Build history of the part. All positions in model axes, mm. Give positions to 0.01 mm unless a question says otherwise; leave off trailing zeros. Write each loop counter-clockwise with the first axis right and the second up, starting at its lowest first coordinate (ties: lowest second). Pieces come first, ordered by that corner, then holes. Notation, with made-up numbers: (28, -25.5) -> (72, -25.5) arc R8 cw to (72, -20.5) -> close; hole circle Ø5 at (-4.5, 35). An arc over 180 degrees is marked (long way). One line per question, with ' | ' between items. Start each with the question number.
(1) Band-saw the part on A-A, the plane z = 0. Give the cut face in (x, y), and give its area (3 significant figures).
(2) Pin check, flat tips, straight feed: P1, Ø0.9, axis at x = 10, y = 1, coming from the +Z side; P2, Ø0.6, axis at y = 1.5, z = 9, coming from the +X side; P3, Ø1.5, axis at y = 1.5, z = 0, coming from the -X side; P4, Ø1.7, axis at x = -21, z = 32.86, coming from the -Y side. Stop position of each tip, or through.
(3) Band-saw the part on C-C, the plane z = -21. Give the cut face in (x, y).
(4) Band-saw the part on D-D, the plane x = -8.5. Give the cut face in (y, z), and give its area (3 significant figures).
(5) Band-saw the part on B-B, the plane x = -55. Give the cut face in (y, z).
(6) Drill centre lines: probe 1 along X at (y, z) = (0.6, 16); probe 2 along X at (y, z) = (1.6, -18); probe 3 along Z at (x, y) = (31.5, 0.55). Where is each one in solid material? Low to high. Write a range as from..to.
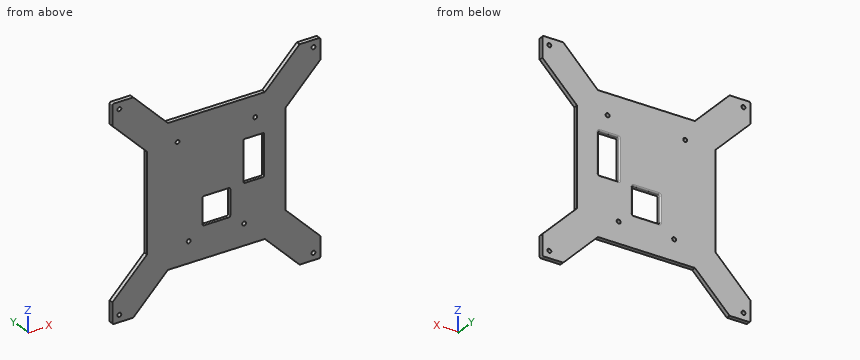
Autodesk Inventor part; units mm, degrees
ref_plane "YZ Plane" through (0, 0, 0) normal (1, 0, 0) x (0, 1, 0)
ref_plane "XZ Plane" through (0, 0, 0) normal (0, 1, 0) x (-1, 0, 0)
ref_plane "XY Plane" through (0, 0, 0) normal (0, 0, 1) x (1, 0, 0)
sketch "Sketch2" plane through (0, 0, 0) normal (0, 1, 0) x (-1, 0, 0)
  line L0 (67.9954, 72.8645) -> (-82.0046, 72.8645)
  line L1 (-82.0046, 72.8645) -> (-82.0046, -77.1355)
  line L2 (-82.0046, -77.1355) -> (67.9954, -77.1355)
  line L3 (67.9954, -77.1355) -> (67.9954, 72.8645)
  circle A0 centre (62.9954, 67.8645) radius 1.4
  line L4 (67.9954, -2.1355) -> (-82.0046, -2.1355)
  line L5 (-7.0046, 72.8645) -> (-7.0046, -77.1355)
  circle A1 centre (62.9954, -72.1355) radius 1.4
  circle A2 centre (-77.0046, 67.8645) radius 1.4
  circle A3 centre (-77.0046, -72.1355) radius 1.4
  point P0 (0, 0)
  dimension "d0" = 150
  dimension "d1" = 150
  dimension "d2" = 5
  dimension "d3" = 5
  dimension "d43" = 2.8
extrude "Extrusion1" add sketch "Sketch2" along normal blind 3
sketch "Sketch4" plane through (0, 3, 0) normal (0, 1, 0) x (1, 0, 0)
  line L0 (-12.9954, 37.1355) -> (27.0046, 37.1355)
  line L1 (27.0046, 37.1355) -> (35.0046, -32.8645)
  line L2 (35.0046, -32.8645) -> (-20.9954, -32.8645)
  line L3 (-20.9954, -32.8645) -> (-12.9954, 37.1355)
  line L4 (7.0046, 37.1355) -> (7.0046, -32.8645)
  line L5 (82.0046, -72.8645) -> (82.0046, 77.1355)
  line L6 (-16.9954, 2.1355) -> (31.0046, 2.1355)
  line L7 (82.0046, 77.1355) -> (-67.9954, 77.1355)
  circle A0 centre (-12.9954, 37.1355) radius 1.4
  circle A1 centre (27.0046, 37.1355) radius 1.4
  circle A2 centre (35.0046, -32.8645) radius 1.4
  circle A3 centre (-20.9954, -32.8645) radius 1.4
  line L8 (26.5046, 9.6355) -> (41.5046, 9.6355)
  line L9 (41.5046, 9.6355) -> (41.5046, -20.3645)
  line L10 (41.5046, -20.3645) -> (26.5046, -20.3645)
  line L11 (26.5046, -20.3645) -> (26.5046, 9.6355)
  line L12 (26.5046, -5.3645) -> (41.5046, -5.3645)
  line L13 (34.0046, 9.6355) -> (34.0046, -20.3645)
  line L14 (-2.9954, 29.6355) -> (17.0046, 29.6355)
  line L15 (17.0046, 29.6355) -> (17.0046, 9.6355)
  line L16 (17.0046, 9.6355) -> (-2.9954, 9.6355)
  line L17 (-2.9954, 9.6355) -> (-2.9954, 29.6355)
  point P0 (0, 0)
  dimension "d17" = 40
  dimension "d18" = 56
  dimension "d19" = 75
  dimension "d20" = 75
  dimension "d21" = 2.8
  dimension "d22" = 2.8
  dimension "d23" = 2.8
  dimension "d24" = 2.8
  dimension "d45" = 70
  dimension "d51" = 15
  dimension "d52" = 30
  dimension "d53" = 27.5
  dimension "d54" = 1
  dimension "d68" = 10
  dimension "d69" = 10
  dimension "d70" = 20
extrude "Extrusion6" cut sketch "Sketch4" against normal through all contours L3 A0 L0 | L0 A0 L3 | A1 L1 L0 | L0 L1 A1 | L14 L15 L16 L4 | L4 L16 L17 L14 | A3 L2 L3 | L3 L2 A3 | L11 L8 L1 L6 | L6 L1 L12 L11 | L8 L13 L12 L1 | A2 L1 L2 | L2 L1 A2 | L12 L1 L10 L11 | L8 L9 L12 L13 | L12 L13 L10 L1 | L12 L9 L10 L13
fillet "Fillet5" radius 1 20 edges at (26.5046, 3, 5.3645) (34.0046, 3, -9.6355) (41.5046, 3, 5.3645) (34.0046, 3, 20.3645) (82.0046, 1.5, 72.8645) (82.0046, 1.5, -77.1355) (-67.9954, 1.5, 72.8645) (-67.9954, 1.5, -77.1355) (41.5046, 1.5, -9.6355) (26.5046, 1.5, -9.6355) (26.5046, 1.5, 20.3645) (41.5046, 1.5, 20.3645) (-2.9954, 3, -19.6355) (7.0046, 3, -29.6355) (-2.9954, 1.5, -29.6355) (7.0046, 3, -9.6355) (17.0046, 3, -19.6355) (17.0046, 1.5, -9.6355) (-2.9954, 1.5, -9.6355) (17.0046, 1.5, -29.6355)
sketch "Sketch8" plane through (0, 3, 0) normal (0, 1, 0) x (1, 0, 0)
  line L0 (-67.9954, 76.1355) -> (-67.9954, -71.8645)
  line L1 (-67.9954, 62.1355) -> (-42.9954, 37.1355)
  line L2 (-42.9954, 37.1355) -> (-42.9954, -32.8645)
  line L3 (-42.9954, -32.8645) -> (-67.9954, -57.8645)
  line L4 (81.0046, 77.1355) -> (-66.9954, 77.1355)
  line L5 (7.0046, 77.1355) -> (7.0046, -72.8645)
  line L6 (-66.9954, -72.8645) -> (81.0046, -72.8645)
  line L7 (82.0046, 62.1355) -> (57.0046, 37.1355)
  line L8 (57.0046, 37.1355) -> (57.0046, -32.8645)
  line L9 (57.0046, -32.8645) -> (82.0046, -57.8645)
  line L10 (-52.9954, 77.1355) -> (-27.9954, 52.1355)
  line L11 (-27.9954, 52.1355) -> (42.0046, 52.1355)
  line L12 (42.0046, 52.1355) -> (67.0046, 77.1355)
  line L13 (-52.9954, -72.8645) -> (-27.9954, -47.8645)
  line L14 (-27.9954, -47.8645) -> (42.0046, -47.8645)
  line L15 (42.0046, -47.8645) -> (67.0046, -72.8645)
  line L16 (82.0046, -71.8645) -> (82.0046, 76.1355)
  point P0 (0, 0)
  dimension "d56" = 25
  dimension "d57" = 15
  dimension "d58" = 15
  dimension "d59" = 25
  dimension "d60" = 25
  dimension "d61" = 15
  dimension "d62" = 15
  dimension "d63" = 15
  dimension "d64" = 25
  dimension "d65" = 25
extrude "Extrusion7" cut sketch "Sketch8" against normal through all
equation "\"d1\" = d0"
equation "\"d22\" = d21"
equation "\"d23\" = d21"
equation "\"d24\" = d21"
properties part number "agv_nano_base"
Results:
1) outline: (-43, 0) -> (26.5, 0) -> (26.5, 2) arc R1 ccw to (25.5, 3) -> (-43, 3) -> close; (41.5, 0) -> (57, 0) -> (57, 3) -> (42.5, 3) arc R1 ccw to (41.5, 2) -> close | area: 255 mm²
2) P1: stops at z = 47.86 | P2: stops at x = 57 | P3: stops at x = -43 | P4: passes through
3) outline: (-43, 0) -> (-3, 0) -> (-3, 2) arc R1 ccw to (-4, 3) -> (-43, 3) -> close; (17, 0) -> (57, 0) -> (57, 3) -> (18, 3) arc R1 ccw to (17, 2) -> close
4) outline: (0, -52.14) -> (3, -52.14) -> (3, 47.86) -> (0, 47.86) -> close | area: 300 mm²
5) outline: (0, -77.14) -> (3, -77.14) -> (3, -49.14) -> (0, -49.14) -> close; (0, 44.87) -> (3, 44.87) -> (3, 72.86) -> (0, 72.86) -> close
6) probe 1: x = -43..26.5, 41.5..57 | probe 2: x = -43..-3, 17..57 | probe 3: z = -52.14..-9.64, 20.36..47.86
